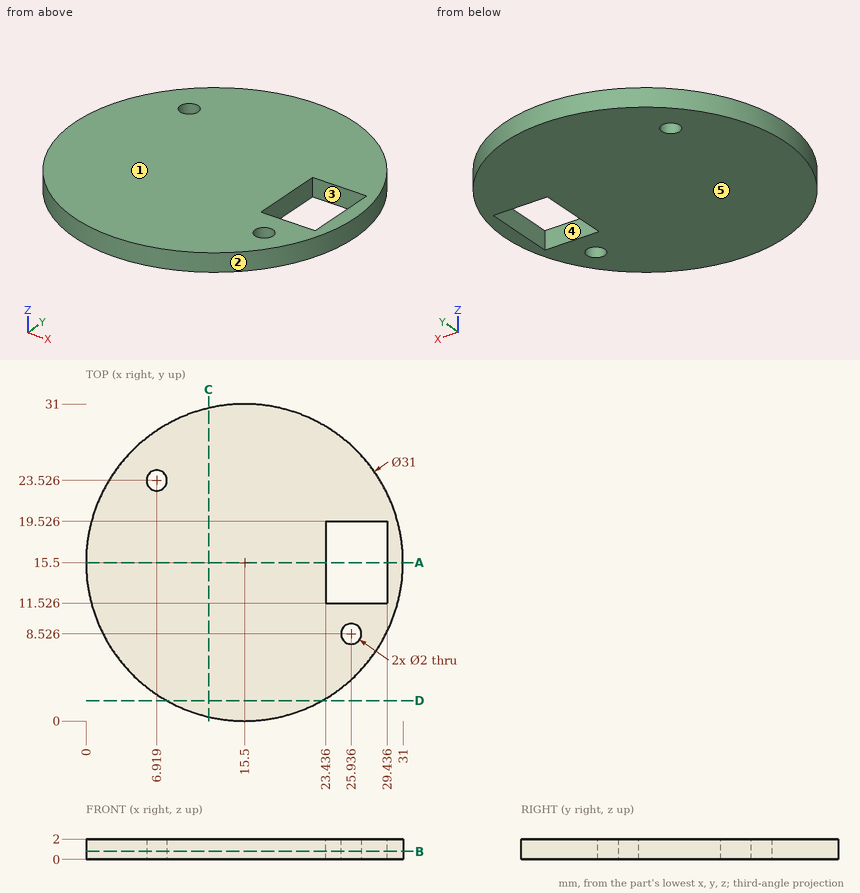
Verification items for this drawing (mm, ordinates from the low corner). A direction names the side the tool comes from. Give positions to 0.01 mm unless a question says otherwise; leave off trailing zeros. Loops run counter-clockwise (first coordinate to the right, second up) from the corner with the lowest first, then second, coordinate; pieces in that order, holes last. Notation, with made-up numbers: M 47.5,19.25 L 85.5,19.25 A32 ccw 85.5,55.25 Z; hole C 66.25,63.5 d9. An arc over 180 degrees is marked long. Write each question's results on one line, items separated by ' | '.
1) Tool access check on the marked faces 4 and 5. Record the directions out of +Z, -Z, +X, -X, +Y, -Y that give a thin tool (end or side, any length) a straight path to the whole face; none if there is none.
Answers follow:
face 4: +Z, -Z | face 5: -Z, +X, -X, +Y, -Y
2) Section check A-A, the plane y = 15.5. Record the boundary of the cut face in (x, z).
Answers follow:
outline: M 0,0 L 23.44,0 L 23.44,2 L 0,2 Z; M 29.44,0 L 31,0 L 31,2 L 29.44,2 Z
3) Thickness scan on line 1 (Y direction, x = 23.5, z = 0.4) (1 decimal); line 2 (X direction, y = 8.5, z = 1.1) (1 decimal); line 3 (X direction, y = 17, z = 0.8). Record the ranges inside material, lowest first.
Answers follow:
line 1: 2.2 to 11.5, 19.5 to 28.8 | line 2: 1.7 to 24.9, 26.9 to 29.3 | line 3: 0.07 to 23.44, 29.44 to 30.93
4) Section check B-B, the plane z = 0.8. Record the boundary of the cut face in (x, y).
Answers follow:
outline: C 15.5,15.5 d31; hole C 6.92,23.53 d2; hole M 23.44,11.53 L 29.44,11.53 L 29.44,19.53 L 23.44,19.53 Z; hole C 25.94,8.53 d2
5) Gauge pin test, flat ends, axial feed: pin 1 (0.6 mm diameter, centred on y = 16.5, z = 1, fed in from +X); pin 2 (1 mm diameter, centred on x = 27.5, z = 1, fed in from -Y). Record the tip position at first contact, or that the pin passes through.
Answers follow:
pin 1: x = 30.98 | pin 2: y = 5.11
6) Release check for a two-part mould opening along Y. For the marked faces 1, 2 and 3 record: +Y half, -Y half, draft (parallel to the pull), parting line (faces both ways), or undercut.
Answers follow:
face 1: draft | face 2: parting line | face 3: undercut
7) Section check C-C, the plane x = 12. Record the boundary of the cut face in (y, z).
Answers follow:
outline: M 0.4,0 L 30.6,0 L 30.6,2 L 0.4,2 Z
8) Section check D-D, the plane y = 2. Record the boundary of the cut face in (x, z).
Answers follow:
outline: M 7.88,0 L 23.12,0 L 23.12,2 L 7.88,2 Z
